```python
from build123d import *

# Parameters (mm, degrees)
BOSS_EXTRUDE1_DEPTH      = 28.575
BOSS_EXTRUDE1_DEPTH_BACK = 28.575
SKETCH2_R                = 37.1475
CUT_EXTRUDE1_DEPTH       = 152.764361406
CUT_EXTRUDE2_DEPTH       = 152.764361406


with BuildPart() as part:
    # Sketch1 → Boss-Extrude1 (new, two sides: drawn at the far end of the back side and taken through both)
    with BuildSketch(Plane(origin=(0, 0, 0), x_dir=(1, 0, 0), z_dir=(0, 1, 0)).offset(-BOSS_EXTRUDE1_DEPTH_BACK)):
        with BuildLine():
            Line((-58.7375, -56.215922718), (-36.318524201, -108.376210733))
            ThreePointArc((-36.318524201, -108.376210733), (-32.806864724, -112.569580799), (-27.567594628, -114.13998))
            Line((-27.567594628, -114.13998), (27.567594628, -114.13998))
            ThreePointArc((27.567594628, -114.13998), (32.806864724, -112.569580799), (36.318524201, -108.376210733))
            Line((36.318524201, -108.376210733), (58.7375, -56.215922718))
            Line((58.7375, -56.215922718), (58.7375, -54.665315944))
            ThreePointArc((58.7375, -54.665315944), (60.229196479, -49.547537174), (64.237061057, -46.032734272))
            Line((64.237061057, -46.032734272), (78.421163742, -39.418578566))
            ThreePointArc((78.421163742, -39.418578566), (81.09307346, -37.075376632), (82.087537779, -33.663524119))
            Line((82.087537779, -33.663524119), (82.087537779, -24.620694942))
            ThreePointArc((82.087537779, -24.620694942), (81.383346428, -21.714263332), (79.426956769, -19.452456605))
            Line((79.426956769, -19.452456605), (62.728014827, -7.531684093))
            ThreePointArc((62.728014827, -7.531684093), (59.800488167, -4.152656806), (58.737193082, 0.189881775))
            ThreePointArc((58.737193082, 0.189881775), (58.584774766, 4.232974359), (58.154386408, 8.255982544))
            Line((58.154386408, 8.255982544), (57.969746696, 9.5565678))
            ThreePointArc((57.969746696, 9.5565678), (59.08262132, 15.536896429), (63.58784972, 19.624161713))
            Line((63.58784972, 19.624161713), (78.279096456, 26.040632326))
            ThreePointArc((78.279096456, 26.040632326), (81.050794671, 28.382496216), (82.087537779, 31.859822947))
            Line((82.087537779, 31.859822947), (82.087537779, 37.284206824))
            ThreePointArc((82.087537779, 37.284206824), (81.09307346, 40.696059337), (78.421163742, 43.039261272))
            Line((78.421163742, 43.039261272), (56.108767451, 53.443702534))
            ThreePointArc((56.108767451, 53.443702534), (52.481431722, 56.405246839), (50.703765355, 60.737476226))
            Line((50.703765355, 60.737476226), (45.968035191, 94.095526633))
            ThreePointArc((45.968035191, 94.095526633), (40.657193823, 103.852471221), (30.25063346, 107.73918))
            Line((30.25063346, 107.73918), (-32.2469722, 107.73918))
            ThreePointArc((-32.2469722, 107.73918), (-41.44482588, 104.803079207), (-47.240370837, 97.080847739))
            Line((-47.240370837, 97.080847739), (-58.7375, 64.036565575))
            Line((-58.7375, 64.036565575), (-58.7375, -56.215922718))
        make_face()
    extrude(amount=BOSS_EXTRUDE1_DEPTH + BOSS_EXTRUDE1_DEPTH_BACK)

    # Sketch2 → Cut-Extrude1 (cut, through all)
    with BuildSketch(Plane(origin=(0, 28.575, 0), x_dir=(1, 0, 0), z_dir=(0, 1, 0))):
        with Locations(Location((0, 0, 0), (0, 0, 270))):
            Circle(SKETCH2_R)
    extrude(amount=-CUT_EXTRUDE1_DEPTH, mode=Mode.SUBTRACT)

    # Sketch5 → Cut-Extrude2 (cut, through all)
    with BuildSketch(Plane.XZ.offset(28.575)):
        with BuildLine():
            Line((-25.4, -86.31428), (25.4, -86.31428))
            ThreePointArc((25.4, -86.31428), (29.3751, -82.33918), (25.4, -78.36408))
            Line((25.4, -78.36408), (-25.4, -78.36408))
            ThreePointArc((-25.4, -78.36408), (-29.3751, -82.33918), (-25.4, -86.31428))
        make_face()
    extrude(amount=-CUT_EXTRUDE2_DEPTH, mode=Mode.SUBTRACT)


solid = part.part
```
Here's how the part is built. I have some questions about the finished solid (model axes, mm). A direction names the side the tool comes from. Coordinates: 2 decimals unless noted, no trailing zeros. Order: outer loops, then holes, each group sorted by start corner. A loop starts at its lowest first (then second) coordinate and runs counter-clockwise, first axis right, second up. Notation, with made-up numbers: (33, -9.75) -> (76, -9.75) arc R18 ccw to (76, -0.75) -> close; hole circle Ø2 at (77, -6). An arc over 180 degrees is marked (long way). Return JSON: item names as keys, results as strings.
1) If we section it at C-C on y = -1.5: State how many separate pieces and enclosed holes the cut face has, plus the area to 3 significant figures.
Conclusion:
{"separate pieces": "1", "enclosed holes": "2", "area": "20,100 mm²"}
2) If we section it at A-A on x = 0: List the corners of the cut face in (y, z) for me (1 decimal).
Conclusion:
{"outline": "(-28.6, -107.7) -> (28.6, -107.7) -> (28.6, -86.3) -> (-28.6, -86.3) -> close; (-28.6, -78.4) -> (28.6, -78.4) -> (28.6, -37.1) -> (-28.6, -37.1) -> close; (-28.6, 37.1) -> (28.6, 37.1) -> (28.6, 114.1) -> (-28.6, 114.1) -> close"}
3) I'm going to push flat-ended pins straight in: P1, Ø0.8, axis at y = 3, z = 55.5, coming from the +X side; P2, Ø10, axis at x = -34.5, y = -19.5, coming from the +Z side. Where does each tip first touch, or does it pass through?
Conclusion:
{"P1": "stops at x = 58.74", "P2": "stops at z = 113.94"}
4) Thinking about a two-plate mould opening in X: for faces 4 (the cylindrical face through (-29.374, -0.4, -82.252)), 5 (the flat face through (71.194, -0.4, 13.576)), 6 (the flat face through (42, 28.575, 2)), which applies, +X half, -X half, draft (parallel to the pull), parting line (faces both ways), or undercut?
Conclusion:
{"face 4": "undercut", "face 5": "+X half", "face 6": "draft"}
5) If I drill on probe 1 along X at (y, z) = (-1, 0); probe 2 along Z at (x, y) = (-7.5, 7); probe 3 along Z at (x, y) = (-12.5, -4), over which ranges is the centre line in solid material (lowest first)?
Conclusion:
{"probe 1": "x = -58.74 to -37.15, 37.15 to 58.74", "probe 2": "z = -107.74 to -86.31, -78.36 to -36.38, 36.38 to 114.14", "probe 3": "z = -107.74 to -86.31, -78.36 to -34.98, 34.98 to 114.14"}
6) If we section it at D-D on z = -67: List the corners of the cut face in (x, y) for me (3 decimals).
Conclusion:
{"outline": "(-57.706, -28.575) -> (49.815, -28.575) -> (49.815, 28.575) -> (-57.706, 28.575) -> close"}
7) If we section it at B-B on z = 12.5: List the corners of the cut face in (x, y) for me (1 decimal).
Conclusion:
{"outline": "(-58.7, -28.6) -> (-35, -28.6) -> (-35, 28.6) -> (-58.7, 28.6) -> close; (35, -28.6) -> (69.7, -28.6) -> (69.7, 28.6) -> (35, 28.6) -> close"}
8) On a 3-axis mill with a long thin cutter (end or side, diameter ignored), from which of +Z, -Z, +X, -X, +Y, -Y can I reach the whole of each face in a straight line? I mean faces 1 (the flat face through (0, 0, -78.364)), 2 (the flat face through (0, 0, 114.14)), 3 (the cylindrical face through (59.83, -0.4, 4.21)). Say none if no direction works.
Conclusion:
{"face 1": "+Y, -Y", "face 2": "+Z, +X, -X, +Y, -Y", "face 3": "+X, +Y, -Y"}
